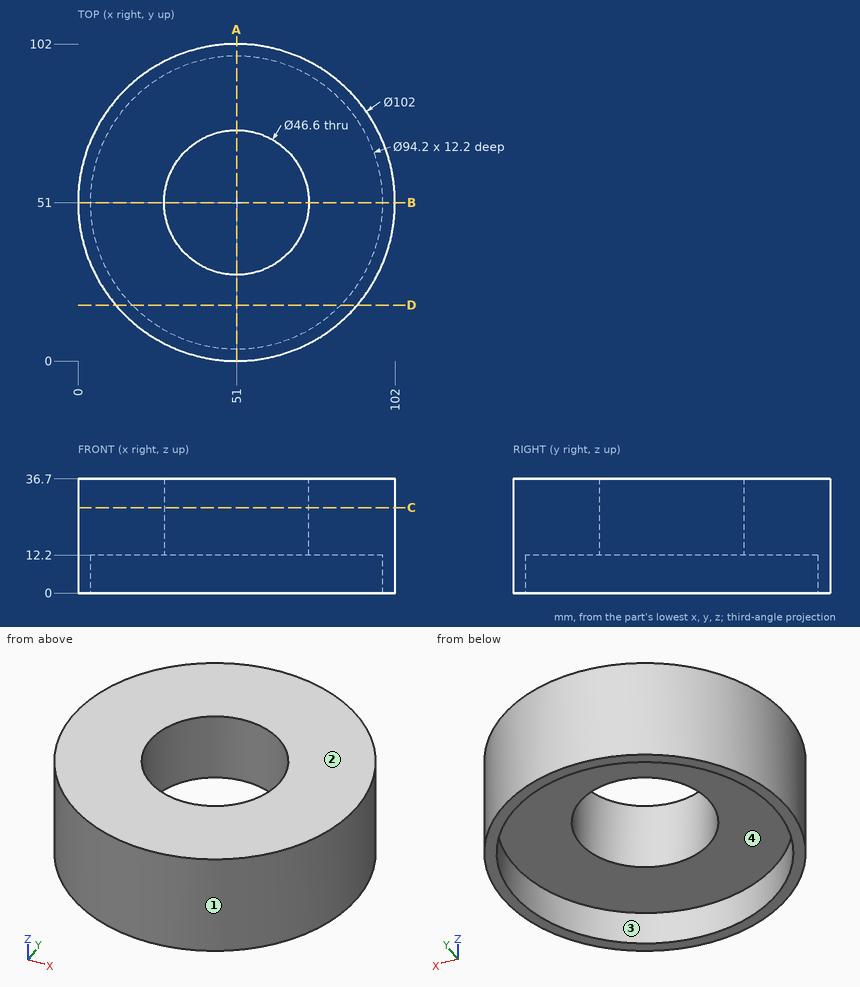
Here's the drawing with two shaded views (mm, measured from the low corner). I have some questions. Give positions to 0.01 mm unless a question says otherwise; leave off trailing zeros. Loops run counter-clockwise (first coordinate to the right, second up) from the corner with the lowest first, then second, coordinate; pieces in that order, holes last. Notation, with made-up numbers: (75.5, 46.25) - (95.5, 46.25) arc R24 ccw to (95.5, 62.25) - close; hole circle Ø6 at (52, -38). An arc over 180 degrees is marked (long way). Return JSON: item names as keys, results as strings.
1. We'd pull the mould along X, two halves only. Please class the marked faces 1, 2, 3 and 4: +X half, -X half, draft (parallel to the pull), parting line (faces both ways), or undercut.
Output values:
{"face 1": "parting line", "face 2": "draft", "face 3": "undercut", "face 4": "undercut"}
2. I want a section at A-A on x = 51. Please give me the cut outline in (y, z).
Output values:
{"outline": "(0, 0) - (3.9, 0) - (3.9, 12.2) - (27.7, 12.2) - (27.7, 36.7) - (0, 36.7) - close; (74.3, 12.2) - (98.1, 12.2) - (98.1, 0) - (102, 0) - (102, 36.7) - (74.3, 36.7) - close"}
3. If I drill on line 1 (Y direction, x = 51, z = 3.5); line 2 (Y direction, x = 51, z = 18.25), over which ranges is the centre line in solid material (lowest first)?
Output values:
{"line 1": "y = 0 to 3.9, 98.1 to 102", "line 2": "y = 0 to 27.7, 74.3 to 102"}
4. I'm going to push flat-ended pins straight in: pin 1 Ø3 at (y, z) = (31.5, 22) entering from +X; pin 2 Ø6 at (x, z) = (30.5, 19.5) entering from +Y; pin 3 Ø1 at (y, z) = (74.5, 9) entering from -X. Where does each tip first touch, or does it pass through?
Output values:
{"pin 1": "stops at x = 98.72", "pin 2": "stops at y = 98.9", "pin 3": "stops at x = 5.48"}
5. I want a section at C-C on z = 27.5. Please give me the cut outline in (x, y), and give its area (3 significant figures).
Output values:
{"outline": "circle Ø102 at (51, 51); hole circle Ø46.6 at (51, 51)", "area": "6,470 mm²"}
6. I want a section at D-D on y = 18. Please give me the cut outline in (x, z).
Output values:
{"outline": "(12.12, 0) - (17.39, 0) - (17.39, 12.2) - (84.61, 12.2) - (84.61, 0) - (89.88, 0) - (89.88, 36.7) - (12.12, 36.7) - close"}
